```python
from build123d import *

# Parameters (mm, degrees)
PAD_DEPTH       = 400
PAD001_DEPTH    = 240
SKETCH002_W     = 176
SKETCH002_H     = 336
POCKET_DEPTH    = 32.001
PAD002_DEPTH    = 220
SKETCH004_R     = 5.25
POCKET001_DEPTH = 212.001


with BuildPart() as part:
    # Sketch → Pad (new body)
    with BuildSketch(Plane.XZ):
        with BuildLine():
            Line((-120, 0), (-120, 32))
            Line((-120, 32), (120, 32))
            Line((120, 32), (120, 0))
            ThreePointArc((116, 4), (117.171573, 1.171573), (120, 0))
            Line((116, 28), (116, 4))
            Line((-116, 28), (116, 28))
            Line((-116, 4), (-116, 28))
            ThreePointArc((-120, 0), (-117.171573, 1.171573), (-116, 4))
        make_face()
    extrude(amount=PAD_DEPTH)

    # Sketch001 (on Face4 of Pad) → Pad001 (join)
    with BuildSketch(Plane(origin=(120, 0, 0), x_dir=(0, 0, 1), z_dir=(1, 0, 0))):
        with BuildLine():
            Line((32, 400), (0, 400))
            ThreePointArc((0, 400), (1.171573, 397.171573), (4, 396))
            Line((4, 396), (32, 396))
            Line((32, 396), (32, 400))
        make_face()
        with BuildLine():
            Line((0, 0), (32, 0))
            Line((32, 0), (32, 4))
            Line((4, 4), (32, 4))
            ThreePointArc((4, 4), (1.171573, 2.828427), (0, 0))
        make_face()
    extrude(amount=-PAD001_DEPTH)

    # Sketch002 (on Face13 of Pad001) → Pocket (cut, through all)
    with BuildSketch(Plane(origin=(0, 0, 32), x_dir=(-1, 0, 0), z_dir=(0, 0, 1))):
        with Locations((0, 200)):
            Rectangle(SKETCH002_W, SKETCH002_H)
    extrude(amount=-POCKET_DEPTH, mode=Mode.SUBTRACT)

    # Sketch003 (on Face13 of Pocket) → Pad002 (join)
    with BuildSketch(Plane(origin=(0, 0, 32), x_dir=(-1, 0, 0), z_dir=(0, 0, 1))):
        with BuildLine():
            Line((88, 216), (88, 184))
            ThreePointArc((88, 184), (90.828427, 185.171573), (92, 188))
            Line((92, 212), (92, 188))
            Line((116, 212), (92, 212))
            ThreePointArc((116, 212), (118.828427, 213.171573), (120, 216))
            Line((88, 216), (120, 216))
        make_face()
        with BuildLine():
            Line((-88, 216), (-120, 216))
            ThreePointArc((-120, 216), (-118.828427, 213.171573), (-116, 212))
            Line((-116, 212), (-92, 212))
            Line((-92, 212), (-92, 188))
            ThreePointArc((-92, 188), (-90.828427, 185.171573), (-88, 184))
            Line((-88, 216), (-88, 184))
        make_face()
    extrude(amount=PAD002_DEPTH)

    # Sketch004 (on Face27 of Pad002) → Pocket001 (cut, through all)
    with BuildSketch(Plane(origin=(92, 0, 0), x_dir=(0, 0, 1), z_dir=(1, 0, 0))):
        with Locations((236, 200)):
            Circle(SKETCH004_R)
    extrude(amount=-POCKET001_DEPTH, mode=Mode.SUBTRACT)


solid = part.part
```
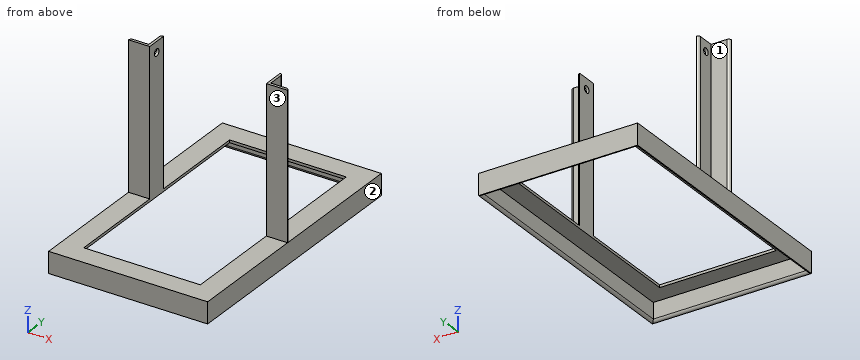
Geometry: final body of the model. Coordinates: model frame, mm. Face numbers are marked on the shaded views. A direction names the side the tool comes from. Give positions to 0.01 mm unless a question says otherwise; leave off trailing zeros. Order: outer loops, then holes, each group sorted by start corner. A loop starts at its lowest first (then second) coordinate and runs counter-clockwise, first axis right, second up. Notation, with made-up numbers: (-3, 83.5) -> (38, 83.5) arc R30 cw to (38, 110.5) -> close; hole circle Ø11 at (56.5, -12). An arc over 180 degrees is marked (long way). Write each question's results on one line, items separated by ' | '. Start each with the question number.
1) Section B-B (z = 236). Return loops of the section in (x, y).
2) Set-up query: the marked faces 1, 2 and 3. Return all of +Z, -Z, +X, -X, +Y, -Y with unobstructed straight access to the full face (end or side cutting, diameter ignored); none if empty.
3) Section D-D (x = -70). Return loops of the section in (y, z).
4) Line query: line 1 (Z direction, x = -90, y = -200); line 2 (X direction, y = -130, z = 12); line 3 (X direction, y = -205, z = 136.5). Output: solid intervals per line, ascending. Write a range as from..to.
5) Section C-C (y = -200). Return loops of the section in (x, z).
6) First-contact query: pin 1 (12 mm diameter, centred on y = -200, z = 236, fed in from +X). Flat tip, straight axial feed; report the tip coordinate or a pass-through.
7) Section A-A (z = 55.5). Return loops of the section in (x, y), then the cut area to 3 significant figures.
Calculated:
1) outline: (-120, -216) -> (-88, -216) -> (-88, -205.25) -> (-92, -205.25) -> (-92, -212) -> (-116, -212) arc R4 ccw to start; (-92, -194.75) -> (-88, -194.75) -> (-88, -184) arc R4 ccw to (-92, -188) -> close; (88, -216) -> (120, -216) arc R4 ccw to (116, -212) -> (92, -212) -> (92, -205.25) -> (88, -205.25) -> close; (88, -194.75) -> (92, -194.75) -> (92, -188) arc R4 ccw to (88, -184) -> close
2) face 1: +Z, -X, +Y | face 2: +Z, -Z, +X, +Y, -Y | face 3: +Z, +X, -X, -Y
3) outline: (-400, 0) arc R4 ccw to (-396, 4) -> (-396, 28) -> (-368, 28) -> (-368, 32) -> (-400, 32) -> close; (-32, 28) -> (-4, 28) -> (-4, 4) arc R4 ccw to (0, 0) -> (0, 32) -> (-32, 32) -> close
4) line 1: 28..230.75, 241.25..252 | line 2: -120..-116, 116..120 | line 3: -92..-88, 88..92
5) outline: (-120, 0) arc R4 ccw to (-116, 4) -> (-116, 28) -> (-88, 28) -> (-88, 230.75) -> (-92, 230.75) -> (-92, 32) -> (-120, 32) -> close; (-92, 241.25) -> (-88, 241.25) -> (-88, 252) -> (-92, 252) -> close; (88, 28) -> (116, 28) -> (116, 4) arc R4 ccw to (120, 0) -> (120, 32) -> (92, 32) -> (92, 230.75) -> (88, 230.75) -> close; (88, 241.25) -> (92, 241.25) -> (92, 252) -> (88, 252) -> close
6) pin 1: x = 92
7) outline: (-120, -216) -> (-88, -216) -> (-88, -184) arc R4 ccw to (-92, -188) -> (-92, -212) -> (-116, -212) arc R4 ccw to start; (88, -216) -> (120, -216) arc R4 ccw to (116, -212) -> (92, -212) -> (92, -188) arc R4 ccw to (88, -184) -> close | area: 466 mm2
